```python
from build123d import *

# Parameters (mm, degrees)
F1_DEPTH = 40.60075
F2_DEPTH = 68.56636
F3_DEPTH = 30.88144
F4_DEPTH = 24.11302


with BuildPart() as f1:
    # F0 (on Front) → F1 (new body)
    with BuildSketch(Plane.XZ):
        with BuildLine():
            Line((63.3510070145, 61.2396271003), (-63.6489929855, 61.2396271003))
            Line((-63.6489929855, 61.2396271003), (-63.6489929855, 10.4396271003))
            Line((-63.6489929855, 10.4396271003), (-6.3833664064, 10.4396271003))
            ThreePointArc((-6.3833664064, 10.4396271003), (-0.080511462, 10.7527853958), (6.2223434824, 10.4396271003))
            Line((6.2223434824, 10.4396271003), (63.3510070145, 10.4396271003))
            Line((63.3510070145, 10.4396271003), (63.3510070145, 61.2396271003))
        make_face()
        Polygon((-63.6489929855, 10.4396271003), (-63.6489929855, 61.2396271003), (-90.8120945096, 61.2396271003), (-90.8120945096, -51.8873035908), (-63.6489929855, -51.8873035908), (-63.6489929855, -51.4030717313), align=None)
        Polygon((85.9697833657, 61.2396271003), (63.3510070145, 61.2396271003), (63.3510070145, 10.4396271003), (63.3510070145, -48.4231859446), (63.3510070145, -51.8873035908), (85.9697833657, -51.8873035908), align=None)
        with BuildLine():
            Line((-6.3833664064, 10.4396271003), (-63.6489929855, 10.4396271003))
            Line((-63.6489929855, 10.4396271003), (-63.6489929855, -51.4030717313))
            ThreePointArc((-63.6489929855, -51.4030717313), (-46.7348870837, -9.6303342951), (-6.3833664064, 10.4396271003))
        make_face()
        with BuildLine():
            Line((63.3510070145, -48.4231859446), (63.3510070145, 10.4396271003))
            Line((63.3510070145, 10.4396271003), (6.2223434824, 10.4396271003))
            ThreePointArc((6.2223434824, 10.4396271003), (45.5476421166, -8.5478399689), (63.3510070145, -48.4231859446))
        make_face()
        with BuildLine():
            ThreePointArc((6.2223434824, 10.4396271003), (-0.080511462, 10.7527853958), (-6.3833664064, 10.4396271003))
            Line((-6.3833664064, 10.4396271003), (6.2223434824, 10.4396271003))
        make_face()
    extrude(amount=F1_DEPTH)

    # F2 (add): faces of the model
    f2_faces = [f1.faces().sort_by_distance(p)[0] for p in [
        (-77.2305437475, -20.300375, -51.8873035908),
        (74.6603951901, -20.300375, -51.8873035908),
    ]]
    extrude(f2_faces, amount=F2_DEPTH)

    # F3 (add): a face of the model
    f3_faces = [f1.faces().sort_by_distance(p)[0] for p in [
        (85.9697833657, -20.300375, -29.6070182453),
    ]]
    extrude(f3_faces, amount=F3_DEPTH)

    # F4 (add): a face of the model
    f4_faces = [f1.faces().sort_by_distance(p)[0] for p in [
        (-90.8120945096, -20.300375, -29.6070182453),
    ]]
    extrude(f4_faces, amount=F4_DEPTH)


solid = f1.part
```
Work out the finished part from the listing and answer in its coordinate system (mm). A direction names the side the tool comes from. Give positions to 0.01 mm unless a question says otherwise; leave off trailing zeros. Loops run counter-clockwise (first coordinate to the right, second up) from the corner with the lowest first, then second, coordinate; pieces in that order, holes last. Notation, with made-up numbers: (-9.5, -15) -> (17.5, -15) arc R29 ccw to (17.5, 15) -> close; hole circle Ø9 at (37, 47). An arc over 180 degrees is marked (long way). Put each result on its own line as item: value. Start each with the question number.
Item 1: Which of the six approach directions +Z, -Z, +X, -X, +Y, -Y give full straight-line access (tool end or side, diameter ignored) to faces 1 (the face through (28, -40.601, 9)), 2 (the face through (63.351, -20, -84))?
Item 2: The part is cut by section D-D (x = 55). Give the vertices of the cut face in (y, z).
Item 3: Find the intervals of material crossed by L1, parallel to X at y = -31.5, z = -96.5; L2, parallel to X at y = -17.5, z = 2; L3, parallel to Z at x = 36, y = -2, in increasing order. Write a range as [from, to].
Item 4: The part is cut by section B-B (y = -37). Give the vertices of the cut face in (x, z), then the cut area to 3 significant figures.
Item 5: Each of these flat-tipped pins is pushed along its axis until it touches: P1, Ø12, axis at x = -45, z = -5, coming from the +Y side; P2, Ø2, axis at x = -41, y = -19, coming from the -Z side; P3, Ø14, axis at x = -0.5, y = -30, coming from the -Z side; P4, Ø8, axis at x = 48, y = -27.5, coming from the -Z side. Where does it stop, or does it pass through?
Item 6: The part is cut by section A-A (z = -82). Give the vertices of the cut face in (x, y).
Item 7: The mould has two halves that part along X. Classify faces 3 (the face through (-63.649, -20, -85)), 4 (the face through (116.851, -20, -31)), 5 (the face through (90, -20, -120.454)): released by +X, released by -X, zero draft, split by the parting line, or undercut.
Item 8: The part is cut by section C-C (z = -8.5). Give the vertices of the cut face in (x, y).
Answers below:
1. face 1: +Z, -Z, +X, -X, -Y
1. face 2: -Z, +Y, -Y
2. outline: (-40.6, -21.06) -> (0, -21.06) -> (0, 61.24) -> (-40.6, 61.24) -> close
3. L1: [-114.93, -63.65], [63.35, 116.85]
3. L2: [-114.93, -32.27], [32.11, 116.85]
3. L3: [-0.48, 61.24]
4. outline: (-114.93, -120.45) -> (-63.65, -120.45) -> (-63.65, -51.4) arc R63.58 cw to (-6.38, 10.44) -> (6.22, 10.44) arc R63.58 cw to (63.35, -48.42) -> (63.35, -120.45) -> (116.85, -120.45) -> (116.85, 61.24) -> (-114.93, 61.24) -> close
4. area: 27,200 mm2
5. P1: y = 0
5. P2: z = -5.02
5. P3: z = 10.32
5. P4: z = -16.35
6. outline: (-114.93, -40.6) -> (-63.65, -40.6) -> (-63.65, 0) -> (-114.93, 0) -> close; (63.35, -40.6) -> (116.85, -40.6) -> (116.85, 0) -> (63.35, 0) -> close
7. face 3: undercut
7. face 4: released by +X
7. face 5: zero draft
8. outline: (-114.93, -40.6) -> (-45.66, -40.6) -> (-45.66, 0) -> (-114.93, 0) -> close; (45.5, -40.6) -> (116.85, -40.6) -> (116.85, 0) -> (45.5, 0) -> close
